Read the model definition and answer for the solid it produces. Units are mm, in the model's axes. Round coordinates to 2 decimals unless told otherwise and drop trailing zeros. Write each loop counter-clockwise with the first axis right and the second up, starting at its lowest first coordinate (ties: lowest second). Pieces come first, ordered by that corner, then holes. Notation, with made-up numbers: (64, 10.5) - (89, 10.5) arc R22 ccw to (89, 19.5) - close; hole circle Ø11 at (-40, -34.5). An arc over 180 degrees is marked (long way). One line per item, written item: value. Start each with the question number.
(1) Flat-ended cylindrical pins translate along their axes: pin 1 Ø2 at (y, z) = (13, -7) entering from +X; pin 2 Ø3 at (x, y) = (11.5, 11) entering from +Z; pin 3 Ø2 at (y, z) = (8, -4.5) entering from +X. Find the tip coordinate at first contact, or state that the pin passes through.
(2) The mould has two halves that part along X. Classify faces 1 (the face through (-12.76, 8.53, -7.5)), 2 (the face through (0, 9, -14.8)), 3 (the face through (-9.76, 8.53, -2.17)): +X half, -X half, draft (parallel to the pull), parting line (faces both ways), or undercut.
(3) A cutting plane is placed at A-A, the plane y = 16.25. Determine the outline of the cut face in (x, z), plus the area to 3 significant figures.
(4) A cutting plane is placed at B-B, the plane y = 10.75. Determine the outline of the cut face in (x, z).
(5) Find the intervals of material crossed by L1, parallel to X at y = 6.5, z = -2.25; L2, parallel to X at y = 11.75, z = -7.25; L3, parallel to Z at x = -3.5, y = 2, in increasing order.
from build123d import *

# Parameters (mm, degrees)
SKETCH_1_R      = 10
EXTRUDE_1_DEPTH = 17.3


with BuildPart() as part:
    # 草图1 → 凸台-拉伸1 (new body)
    with BuildSketch(Plane(origin=(0, 0, 0), x_dir=(1, 0, 0), z_dir=(0, 1, 0))):
        Polygon((17.089567968, 0), (8.544783984, 14.8), (-8.544783984, 14.8), (-17.089567968, 0), (-8.544783984, -14.8), (8.544783984, -14.8), align=None)
        with Locations(Location((0, 0, 0), (0, 0, 270))):
            Circle(SKETCH_1_R, mode=Mode.SUBTRACT)
    extrude(amount=EXTRUDE_1_DEPTH)

    # 草图3 → 切除-旋转4 (revolve, cut)
    with BuildSketch(Plane(origin=(0, 0, 0), x_dir=(-0.5000000000000007, 0, -0.8660254037844383), z_dir=(0.8660254037844383, 0, -0.5000000000000007))):
        with BuildLine():
            Line((-14.8, 17.3), (-14.8, 17.928720004))
            Line((-14.8, 17.928720004), (-17.799472335, 17.928720004))
            Line((-17.799472335, 17.928720004), (-17.799472335, 15.010432032))
            Line((-17.799472335, 15.010432032), (-17.089567968, 15.010432032))
            ThreePointArc((-17.089567968, 15.010432032), (-16.301064282, 16.511496314), (-14.8, 17.3))
        make_face()
        with BuildLine():
            Line((-17.799472335, 2.289567968), (-17.089567968, 2.289567968))
            ThreePointArc((-17.089567968, 2.289567968), (-16.301064282, 0.788503686), (-14.8, 0))
            Line((-14.8, 0), (-14.8, -0.628720004))
            Line((-14.8, -0.628720004), (-17.799472335, -0.628720004))
            Line((-17.799472335, -0.628720004), (-17.799472335, 2.289567968))
        make_face()
    revolve(axis=Axis((0, 0, 0), (0, 1, 0)), mode=Mode.SUBTRACT)


solid = part.part
Here are the results:
1. pin 1: x = 13.63
1. pin 2: z = 12.28
1. pin 3: x = 15.07
2. face 1: -X half
2. face 2: draft
2. face 3: undercut
3. outline: (-16.5, -1.02) - (-9.13, -13.78) arc R16.53 ccw to (-7.37, -14.8) - (7.37, -14.8) arc R16.53 ccw to (9.13, -13.78) - (16.5, -1.02) arc R16.53 ccw to (16.5, 1.02) - (9.13, 13.78) arc R16.53 ccw to (7.37, 14.8) - (-7.37, 14.8) arc R16.53 ccw to (-9.13, 13.78) - (-16.5, 1.02) arc R16.53 ccw to start; hole circle Ø20 at (0, 0)
3. area: 441 mm²
4. outline: (-17.09, 0) - (-8.54, -14.8) - (8.54, -14.8) - (17.09, 0) - (8.54, 14.8) - (-8.54, 14.8) - close; hole circle Ø20 at (0, 0)
5. L1: -15.79 to -9.74, 9.74 to 15.79
5. L2: -12.9 to -6.89, 6.89 to 12.9
5. L3: -14.8 to -9.37, 9.37 to 14.8
